CAD build for the part. Positions are in the model's coordinates, mm. A direction names the side the tool comes from. Round coordinates to 2 decimals unless told otherwise and drop trailing zeros. Order: outer loops, then holes, each group sorted by start corner. A loop starts at its lowest first (then second) coordinate and runs counter-clockwise, first axis right, second up. Notation, with made-up numbers: (-13.75, -5.5) -> (17.25, -5.5) arc R20 cw to (17.25, 23.5) -> close; hole circle Ø6 at (35.25, 60.25). An arc over 180 degrees is marked (long way). Return JSON: item names as keys, results as strings. Group by question number.
Q1. Cut at A-A (z = -5.5). Write the cut outline in (x, y).
Q2. Cut at C-C (x = 17). Write the cut outline in (y, z), then the cut area to 3 significant figures.
Q3. Flat gauge pins, fed straight in: pin 1 (1 mm diameter, centred on x = 1, z = -48.5, fed in from -Y); pin 2 (3 mm diameter, centred on x = -9.5, y = 28.5, fed in from +Z). Where does each tip first touch, or does it go through?
Q4. Mould opens along Z. For faces 1 (the flat face through (-32, 1, -24)), 2 (the flat face through (-33, 1, 0)), 3 (the flat face through (34.5, -44, -25)) say: +Z half, -Z half, draft (parallel to the pull), parting line (faces both ways), or undercut.
Q5. Probe line 1 along X through (y, z) = (-8, -31); line 2 along Z through (x, y) = (17.5, -22). List the from-to ranges inside material, lowest first.
Q6. Which spindle directions (+Z, -Z, +X, -X, +Y, -Y) get a long thin tool onto all of the face, cutting with end or side? Do faces 4 (the flat face through (33, 44, -23)), 5 (the flat face through (35, 1, -25)), 6 (the flat face through (-34, -44, -23)). Say none if no direction does.
Q7. Cut at B-B (y = -7). Write the cut outline in (x, z), then the cut area to 3 significant figures.
from build123d import *

# Parameters (mm, degrees)
BOSS_EXTRUDE1_DEPTH = 45
SKETCH2_W           = 2
SKETCH2_H           = 4
SKETCH2_W_2         = 4
SKETCH2_H_2         = 2
CUT_EXTRUDE1_DEPTH  = 3


with BuildPart() as part:
    # Sketch1 → Boss-Extrude1 (new, symmetric)
    with BuildSketch(Plane(origin=(0, 0, 0), x_dir=(1, 0, 0), z_dir=(0, 1, 0))):
        Polygon((-35, 0), (-35, 50), (35, 50), (35, 0), (32, 0), (32, 47), (-32, 47), (-32, 0), align=None)
    extrude(amount=BOSS_EXTRUDE1_DEPTH, both=True)

    # Sketch2 → Cut-Extrude1 (cut)
    with BuildSketch(Plane(origin=(0, 45, 0), x_dir=(1, 0, 0), z_dir=(0, 1, 0))):
        with Locations((33.5, 25)):
            Rectangle(SKETCH2_W, SKETCH2_H)
        with Locations((-33.5, 25)):
            Rectangle(SKETCH2_W, SKETCH2_H)
        with Locations((0, 48.5)):
            Rectangle(SKETCH2_W_2, SKETCH2_H_2)
    cut_extrude1 = extrude(amount=-CUT_EXTRUDE1_DEPTH, mode=Mode.SUBTRACT)

    # Mirror1: Cut-Extrude1 across plane
    add(cut_extrude1.mirror(Plane.ZX), mode=Mode.SUBTRACT)


solid = part.part
Solution:
{
 "1": {"outline": "(-35, -45) -> (-32, -45) -> (-32, 45) -> (-35, 45) -> close; (32, -45) -> (35, -45) -> (35, 45) -> (32, 45) -> close"},
 "2": {"outline": "(-45, -50) -> (45, -50) -> (45, -47) -> (-45, -47) -> close", "area": "270 mm²"},
 "3": {"pin 1": "stops at y = -42", "pin 2": "stops at z = -47"},
 "4": {"face 1": "draft", "face 2": "+Z half", "face 3": "undercut"},
 "5": {"line 1": "x = -35 to -32, 32 to 35", "line 2": "z = -50 to -47"},
 "6": {"face 4": "+Y", "face 5": "+Z, -Z, +X, +Y, -Y", "face 6": "-Y"},
 "7": {"outline": "(-35, -50) -> (35, -50) -> (35, 0) -> (32, 0) -> (32, -47) -> (-32, -47) -> (-32, 0) -> (-35, 0) -> close", "area": "492 mm²"}
}
